Geometry check sheet. Reference: the model listing, model coordinates, mm. Coordinates: 2 decimals unless noted, no trailing zeros. Order: outer loops, then holes, each group sorted by start corner. A loop starts at its lowest first (then second) coordinate and runs counter-clockwise, first axis right, second up.
```python
from build123d import *

# Parameters (mm, degrees)
SKETCH_1_R      = 10.2
SKETCH_1_R_2    = 1.5
SKETCH_1_R_3    = 4.2
EXTRUDE_1_DEPTH = 1


with BuildPart() as part:
    # Эскиз1 → Бобышка-Вытянуть1 (new, symmetric)
    with BuildSketch(Plane.XY):
        Circle(SKETCH_1_R)
        with Locations((-6.711696879, -3.875)):
            Circle(SKETCH_1_R_2, mode=Mode.SUBTRACT)
        with Locations((0, 7.75)):
            Circle(SKETCH_1_R_2, mode=Mode.SUBTRACT)
        with Locations((6.711696879, -3.875)):
            Circle(SKETCH_1_R_2, mode=Mode.SUBTRACT)
        Circle(SKETCH_1_R_3, mode=Mode.SUBTRACT)
    extrude(amount=EXTRUDE_1_DEPTH, both=True)


solid = part.part
```
Item 1: Release check for a two-part mould opening along Y. For faces 1 (the face through (-0.1, -4.4, -1)), 2 (the face through (4.707, -9.049, 0.014)), 3 (the face through (4.006, 1.262, -0.014)) record: pulls with the +Y half, pulls with the -Y half, needs draft (parallel to the pull), parting line crosses it, or undercut.
Item 2: Thickness scan on line 1 along Y through (x, z) = (0, -0.2); line 2 along X through (y, z) = (-5.25, 0.9); line 3 along Y through (x, z) = (-7.75, -0.75). Record the ranges inside material, lowest first.
Item 3: Sectioned sample at B-B (y = 0). Record the cut outline in (x, z), and give its area (3 significant figures).
Item 4: Sectioned sample at C-C (y = -5). Record the cut outline in (x, z), and give its area (3 significant figures).
Item 5: Depth check by flat-ended pin: P1, Ø2.5, axis at x = 6.71, y = -3.88, coming from the -Z side. Enter the tip coordinate at first touch or a pass-through.
Item 6: Sectioned sample at D-D (x = 7.25). Record the cut outline in (y, z), and give its area (3 significant figures).
Item 7: Sectioned sample at A-A (x = 0). Record the cut outline in (y, z).
Geometry check:
1. face 1: needs draft
1. face 2: parting line crosses it
1. face 3: undercut
2. line 1: y = -10.2 to -4.2, 4.2 to 6.25, 9.25 to 10.2
2. line 2: x = -8.75 to -7.31, -6.11 to 6.11, 7.31 to 8.75
2. line 3: y = -6.63 to -4.96, -2.79 to 6.63
3. outline: (-10.2, -1) - (-4.2, -1) - (-4.2, 1) - (-10.2, 1) - close; (4.2, -1) - (10.2, -1) - (10.2, 1) - (4.2, 1) - close
3. area: 24.0 mm2
4. outline: (-8.89, -1) - (-7.7, -1) - (-7.7, 1) - (-8.89, 1) - close; (-5.72, -1) - (5.72, -1) - (5.72, 1) - (-5.72, 1) - close; (7.7, -1) - (8.89, -1) - (8.89, 1) - (7.7, 1) - close
4. area: 27.6 mm2
5. P1: passes through
6. outline: (-7.17, -1) - (-5.28, -1) - (-5.28, 1) - (-7.17, 1) - close; (-2.47, -1) - (7.17, -1) - (7.17, 1) - (-2.47, 1) - close
6. area: 23.1 mm2
7. outline: (-10.2, -1) - (-4.2, -1) - (-4.2, 1) - (-10.2, 1) - close; (4.2, -1) - (6.25, -1) - (6.25, 1) - (4.2, 1) - close; (9.25, -1) - (10.2, -1) - (10.2, 1) - (9.25, 1) - close
